```python
from build123d import *

# Parameters (mm, degrees)
SKETCH_3_R          = 2.7
EXTRUDE_2_DEPTH     = 26
SKETCH_5_R          = 5
CUT_EXTRUDE_1_DEPTH = 1
CUT_EXTRUDE_2_DEPTH = 1
CUT_EXTRUDE_3_DEPTH = 24
EXTRUDE_3_DEPTH     = 1
CHAMFER_1_SIZE      = 0.5
SKETCH_9_W          = 21
SKETCH_9_H          = 5.775015532
EXTRUDE_4_DEPTH     = 5
CHAMFER_3_SIZE      = 0.5
EXTRUDE_5_DEPTH     = 10
CHAMFER_4_SIZE      = 2


with BuildPart() as part:
    # Sketch 3 → Extrude 2 (new body)
    with BuildSketch(Plane.XY):
        with BuildLine():
            Line((25.85, 10), (-25.85, 10))
            ThreePointArc((-25.85, 10), (-27.971320344, 9.121320344), (-28.85, 7))
            Line((-28.85, 7), (-28.85, 0))
            Line((-28.85, 0), (-28.85, -12))
            ThreePointArc((-28.85, -12), (-27.971320344, -14.121320344), (-25.85, -15))
            Line((-25.85, -15), (25.85, -15))
            ThreePointArc((25.85, -15), (27.971320344, -14.121320344), (28.85, -12))
            Line((28.85, -12), (28.85, 0))
            Line((28.85, 0), (28.85, 7))
            ThreePointArc((28.85, 7), (27.971320344, 9.121320344), (25.85, 10))
        make_face()
        with Locations(Location((-16.35, 0, 0), (0, 0, 180))):
            Circle(SKETCH_3_R, mode=Mode.SUBTRACT)
        with Locations(Location((16.35, 0, 0), (0, 0, 180))):
            Circle(SKETCH_3_R, mode=Mode.SUBTRACT)
    extrude(amount=EXTRUDE_2_DEPTH)

    # Sketch 5 → Cut-Extrude 1 (cut)
    with BuildSketch(Plane.XY.offset(26)):
        with Locations((-16.35, 0)):
            Circle(SKETCH_5_R)
        with Locations(Location((16.35, 0, 0), (0, 0, 180))):
            Circle(SKETCH_5_R)
    extrude(amount=-CUT_EXTRUDE_1_DEPTH, mode=Mode.SUBTRACT)

    # Sketch 6 → Cut-Extrude 2 (cut)
    with BuildSketch(Plane.XY.offset(26)):
        with BuildLine():
            Line((5, -9.000269215), (-5, -9.000269215))
            add(Edge.make_bspline(
                [(-5, -9.000269215), (-5, -11.500269215), (0, -11.500269215), (5, -11.500269215), (5, -9.000269215)],
                knots=[3.141592654, 3.141592654, 3.141592654, 4.71238898, 4.71238898, 6.283185307, 6.283185307, 6.283185307], degree=2, weights=[1, 0.707106781, 1, 0.707106781, 1]))
        make_face()
        with BuildLine():
            Line((-21.317949192, -9.346410161), (-24.782050808, -7.346410161))
            ThreePointArc((-24.782050808, -7.346410161), (-24.928460969, -6.8), (-24.382050808, -6.653589838))
            Line((-24.382050808, -6.653589838), (-20.917949192, -8.653589838))
            ThreePointArc((-20.917949192, -8.653589838), (-20.771539031, -9.2), (-21.317949192, -9.346410161))
        make_face()
        with BuildLine():
            Line((-17.317949192, -9.346410161), (-20.782050808, -7.346410161))
            ThreePointArc((-20.782050808, -7.346410161), (-20.928460969, -6.8), (-20.382050808, -6.653589838))
            Line((-20.382050808, -6.653589838), (-16.917949192, -8.653589838))
            ThreePointArc((-16.917949192, -8.653589838), (-16.771539031, -9.2), (-17.317949192, -9.346410161))
        make_face()
        with BuildLine():
            Line((-13.317949192, -9.346410161), (-16.782050808, -7.346410161))
            ThreePointArc((-16.782050808, -7.346410161), (-16.928460969, -6.8), (-16.382050808, -6.653589838))
            Line((-16.382050808, -6.653589838), (-12.917949192, -8.653589838))
            ThreePointArc((-12.917949192, -8.653589838), (-12.771539031, -9.2), (-13.317949192, -9.346410161))
        make_face()
        with BuildLine():
            Line((-9.317949192, -9.346410161), (-12.782050808, -7.346410161))
            ThreePointArc((-12.782050808, -7.346410161), (-12.928460969, -6.8), (-12.382050808, -6.653589838))
            Line((-12.382050808, -6.653589838), (-8.917949192, -8.653589838))
            ThreePointArc((-8.917949192, -8.653589838), (-8.771539031, -9.2), (-9.317949192, -9.346410161))
        make_face()
        with BuildLine():
            Line((12.382050808, -9.346410161), (8.917949192, -7.346410161))
            ThreePointArc((8.917949192, -7.346410161), (8.771539031, -6.8), (9.317949192, -6.653589838))
            Line((9.317949192, -6.653589838), (12.782050808, -8.653589838))
            ThreePointArc((12.782050808, -8.653589838), (12.928460969, -9.2), (12.382050808, -9.346410161))
        make_face()
        with BuildLine():
            Line((16.382050808, -9.346410161), (12.917949192, -7.346410161))
            ThreePointArc((12.917949192, -7.346410161), (12.771539031, -6.8), (13.317949192, -6.653589838))
            Line((13.317949192, -6.653589838), (16.782050808, -8.653589838))
            ThreePointArc((16.782050808, -8.653589838), (16.928460969, -9.2), (16.382050808, -9.346410161))
        make_face()
        with BuildLine():
            Line((20.382050808, -9.346410161), (16.917949192, -7.346410161))
            ThreePointArc((16.917949192, -7.346410161), (16.771539031, -6.8), (17.317949192, -6.653589838))
            Line((17.317949192, -6.653589838), (20.782050808, -8.653589838))
            ThreePointArc((20.782050808, -8.653589838), (20.928460969, -9.2), (20.382050808, -9.346410161))
        make_face()
        with BuildLine():
            Line((24.382050808, -9.346410161), (20.917949192, -7.346410161))
            ThreePointArc((20.917949192, -7.346410161), (20.771539031, -6.8), (21.317949192, -6.653589838))
            Line((21.317949192, -6.653589838), (24.782050808, -8.653589838))
            ThreePointArc((24.782050808, -8.653589838), (24.928460969, -9.2), (24.382050808, -9.346410161))
        make_face()
    extrude(amount=-CUT_EXTRUDE_2_DEPTH, mode=Mode.SUBTRACT)

    # Sketch 7 → Cut-Extrude 3 (cut, symmetric)
    with BuildSketch(Plane(origin=(0, 0, 0), x_dir=(0, 0, -1), z_dir=(1, 0, 0))):
        Polygon((0, 8.4), (-1.8, 8.4), (-7.2, 3), (-7.2, -6.8), (-18.2, -6.8), (-18.2, -15), (0, -15), align=None)
    extrude(amount=CUT_EXTRUDE_3_DEPTH, both=True, mode=Mode.SUBTRACT)

    # Sketch 8 → Extrude 3 (add)
    with BuildSketch(Plane.XY):
        Polygon((-24, 2.9), (-28.85, 2.9), (-28.85, -2.875015532), (-24, -2.9), align=None)
        Polygon((28.85, -2.875015532), (24, -2.9), (24, 2.9), (28.85, 2.9), align=None)
    extrude(amount=-EXTRUDE_3_DEPTH)

    # Chamfer 1
    chamfer_1_edges = [part.edges().sort_by_distance(p)[0] for p in [
        (-24, 0, -1),
        (-26.425, -2.887507766, -1),
        (-28.85, 0.012492234, -1),
        (-26.425, 2.9, -1),
        (28.85, 0.012492234, -1),
        (26.425, -2.887507766, -1),
        (24, 0, -1),
        (26.425, 2.9, -1),
    ]]
    chamfer(chamfer_1_edges, length=CHAMFER_1_SIZE)

    # Sketch 9 → Extrude 4 (add)
    with BuildSketch(Plane.ZY.offset(28.85)):
        with Locations((15.5, 0.012492234)):
            Rectangle(SKETCH_9_W, SKETCH_9_H)
    extrude(amount=EXTRUDE_4_DEPTH)

    # Chamfer 3
    chamfer_3_edges = [part.edges().sort_by_distance(p)[0] for p in [
        (27.971320344, -14.121320344, 26),
        (28.85, -2.5, 26),
        (-28.85, -7.437507766, 26),
        (-31.35, 2.9, 26),
        (-31.35, -2.875015532, 26),
        (-33.85, 2.9, 15.5),
        (-33.85, 0.012492234, 5),
        (-33.85, -2.875015532, 15.5),
        (27.971320344, 9.121320344, 26),
        (0, 10, 26),
        (-27.971320344, 9.121320344, 26),
        (-28.85, 4.95, 26),
        (-27.971320344, -14.121320344, 26),
        (0, -15, 26),
    ]]
    chamfer(chamfer_3_edges, length=CHAMFER_3_SIZE)

    # Sketch 10 → Extrude 5 (add, symmetric)
    with BuildSketch(Plane(origin=(0, 0, 0), x_dir=(0, 0, -1), z_dir=(1, 0, 0))):
        Polygon((-7.2, -6.8), (0, -6.8), (0, 8.4), (-1.8, 8.4), (-7.2, 3), align=None)
    extrude(amount=EXTRUDE_5_DEPTH, both=True)

    # Chamfer 4
    chamfer_4_edges = [part.edges().sort_by_distance(p)[0] for p in [
        (-10, -1.9, 7.2),
        (-10, 8.4, 0.9),
        (-10, 5.7, 4.5),
        (10, -1.9, 7.2),
        (10, 8.4, 0.9),
        (10, 5.7, 4.5),
    ]]
    chamfer(chamfer_4_edges, length=CHAMFER_4_SIZE)

    # Sketch 4 → Cut-Revolve 1 (revolve, cut)
    with BuildSketch(Plane(origin=(0, 0, 0), x_dir=(0, 0, -1), z_dir=(1, 0, 0)), mode=Mode.PRIVATE) as cut_revolve_1_sk:
        with BuildLine():
            Line((-13, 10), (-13, -15))
            Line((-13, -15), (-11.4, -15))
            Line((-11.4, -15), (-11.4, 0))
            Line((-11.4, 0), (-8.8, 0))
            ThreePointArc((-8.8, 0), (-5.068620963, 1.38559814), (-3.5, 5.043808085))
            Line((-3.5, 5.043808085), (-3.5, 10))
            Line((-3.5, 10), (-13, 10))
        make_face()
    revolve(cut_revolve_1_sk.sketch.rotate(Axis((0, 10, 13), (0, -1, 0)), 180), axis=Axis((0, 10, 13), (0, -1, 0)), mode=Mode.SUBTRACT)


solid = part.part
```
Geometry check sheet. Reference: the model listing, model coordinates, mm. A direction names the side the tool comes from. Coordinates: 2 decimals unless noted, no trailing zeros. One line per item, written item: value. Start each with the question number.
(1) Depth check by flat-ended pin: pin 1 (14.5 mm diameter, centred on x = 2, z = 5, fed in from -Y); pin 2 (9 mm diameter, centred on x = 1.5, z = 12.5, fed in from +Y); pin 3 (1.5 mm diameter, centred on y = 5, z = 10.5, fed in from -X). Enter the tip coordinate at first touch or a pass-through.
(2) Release check for a two-part mould opening along Y. For faces 6 (the face through (26, 0, -1)), 7 (the face through (15, -8, 25)), 8 (the face through (6, 10, 21)) record: released by +Y, released by -Y, zero draft, split by the parting line, or undercut.
(3) Sectioned sample at A-A, the plane z = 20.25. State how many separate pieces and enclosed holes the cut face has, and give its area (3 significant figures).
(4) Scan lines: line 1 along X through (y, z) = (-5.5, 1.25); line 2 along X through (y, z) = (-7, 0.75); line 3 along X through (y, z) = (-1.5, 9.75) (3 decimals). Record each from-to range of solid material in increasing order. Write a range as [from, to].
(5) Tool access check on faces 1 (the face through (26, -9, 0)), 2 (the face through (27.739, 8.848, 25.858)), 3 (the face through (-11, -1.8, 6.2)), 4 (the face through (10.67, -8.36, 25.51)), 5 (the face through (-26, 0, -1)). Record the directions out of +Z, -Z, +X, -X, +Y, -Y that give a thin tool (end or side, any length) a straight path to the whole face; none if there is none.
Filled sheet:
1. pin 1: y = -6.8
1. pin 2: y = 0.26
1. pin 3: x = -28.85
2. face 6: zero draft
2. face 7: undercut
2. face 8: released by +Y
3. separate pieces: 1
3. enclosed holes: 2
3. area: 1,320 mm²
4. line 1: [-28.85, -24], [-10, 10], [24, 28.85]
4. line 2: [-28.85, -24], [24, 28.85]
4. line 3: [-33.85, -18.595], [-14.105, 14.105], [18.595, 28.85]
5. face 1: -Z, +X, -X, -Y
5. face 2: +Z, +X, +Y
5. face 3: -Z, -Y
5. face 4: +Z
5. face 5: -Z, +X, -X, +Y, -Y
